```python
from build123d import *

# Parameters (mm, degrees)
F0_R     = 50
F1_DEPTH = 20
F2_R     = 47.5
F3_DEPTH = 10
F4_R     = 5
F5_R     = 5
F6_R     = 5
F7_DEPTH = 25


with BuildPart() as f1:
    # F0 (on Right) → F1 (new body)
    with BuildSketch(Plane.YZ):
        with Locations((-0.053118, 0.106767)):
            Circle(F0_R)
    extrude(amount=F1_DEPTH)

    # F2 (on face) → F3 (cut)
    with BuildSketch(Plane(origin=(0, 0, 0), x_dir=(0, -1, 0), z_dir=(-1, 0, 0))):
        Circle(F2_R)
    extrude(amount=-F3_DEPTH, mode=Mode.SUBTRACT)

    # F4
    f4_edges = [f1.edges().sort_by_distance(p)[0] for p in [
        (10, 47.5, 0),
    ]]
    fillet(f4_edges, radius=F4_R)

    # F5
    f5_edges = [f1.edges().sort_by_distance(p)[0] for p in [
        (10, 42.5, 0),
        (20, -50.053118, 0.106767),
    ]]
    fillet(f5_edges, radius=F5_R)

    # F6 (on face) → F7 (cut)
    with BuildSketch(Plane(origin=(10, 0, 0), x_dir=(0, -1, 0), z_dir=(-1, 0, 0))):
        Circle(F6_R)
    extrude(amount=-F7_DEPTH, mode=Mode.SUBTRACT)


solid = f1.part
```
CAD build for the part. Positions are in the model's coordinates, mm. A direction names the side the tool comes from. Give positions to 0.01 mm unless a question says otherwise; leave off trailing zeros. Write each loop counter-clockwise with the first axis right and the second up, starting at its lowest first coordinate (ties: lowest second). Pieces come first, ordered by that corner, then holes. Notation, with made-up numbers: (64, -39) -> (74, -39) arc R10 cw to (74, -21) -> close; hole circle Ø2 at (75, 81.25). An arc over 180 degrees is marked (long way). Write each question's results on one line, items separated by ' | '.
1. Cut at A-A, the plane x = 17.5. Write the cut outline in (y, z), then the cut area to 3 significant figures.
Geometry check:
outline: circle Ø98.66 at (-0.05, 0.11); hole circle Ø10 at (0, 0) | area: 7,570 mm²
2. Two-plate mould, pull along Y, no slides. Class faces 3 (the cylindrical face through (7.395, -36.905, 33.899)), 4 (the flat face through (0, 48, 0)), 5 (the cylindrical face through (14.93, 1.08, -4.88)): pulls with the +Y half, pulls with the -Y half, needs draft (parallel to the pull), parting line crosses it, or undercut.
Geometry check:
face 3: parting line crosses it | face 4: needs draft | face 5: undercut
3. Cut at B-B, the plane x = 12. Write the cut outline in (y, z), then the cut area to 3 significant figures.
Geometry check:
outline: circle Ø100 at (-0.05, 0.11); hole circle Ø10 at (0, 0) | area: 7,780 mm²
4. Which spindle directions (+Z, -Z, +X, -X, +Y, -Y) get a long thin tool onto all of the face, cutting with end or side? Do faces 1 (the flat face through (20, -1, -9)), 2 (the flat face through (10, 1, -9)). Say none if no direction does.
Geometry check:
face 1: +Z, -Z, +X, +Y, -Y | face 2: -X
5. Wall check: probe 1 along Z at (x, y) = (12.5, 0); probe 2 along Z at (x, y) = (1.7, 0); probe 3 along X at (y, z) = (2, -9.5). Give the ranges that are in metal, low to high. Write a range as [from, to].
Geometry check:
probe 1: [-49.89, -5], [5, 50.11] | probe 2: [-49.89, -47.5], [47.5, 50.11] | probe 3: [10, 20]
6. Drop flat-ended pins along their axis: P1, Ø6, axis at x = 3.5, z = 4, coming from the +Y side; P2, Ø4, axis at x = 17, z = 26.5, coming from the +Y side; P3, Ø6, axis at x = 7.5, y = -29, coming from the +Z side. Give the stop position or say it passes through.
Geometry check:
P1: y = 49.94 | P2: y = 43.33 | P3: z = 42.85
